Design review of the part shown in the three views and the two pictorial views. Dimensions are in mm from the part's minimum x, y and z. A direction names the side the tool comes from. Give positions to 0.01 mm unless a question says otherwise; leave off trailing zeros. Loops run counter-clockwise (first coordinate to the right, second up) from the corner with the lowest first, then second, coordinate; pieces in that order, holes last. Notation, with made-up numbers: (79.25, 15) - (93.25, 15) arc R36 cw to (93.25, 49) - close; hole circle Ø11 at (-10, -25.5). An arc over 180 degrees is marked (long way). Return JSON: item names as keys, results as strings. Group by question number.
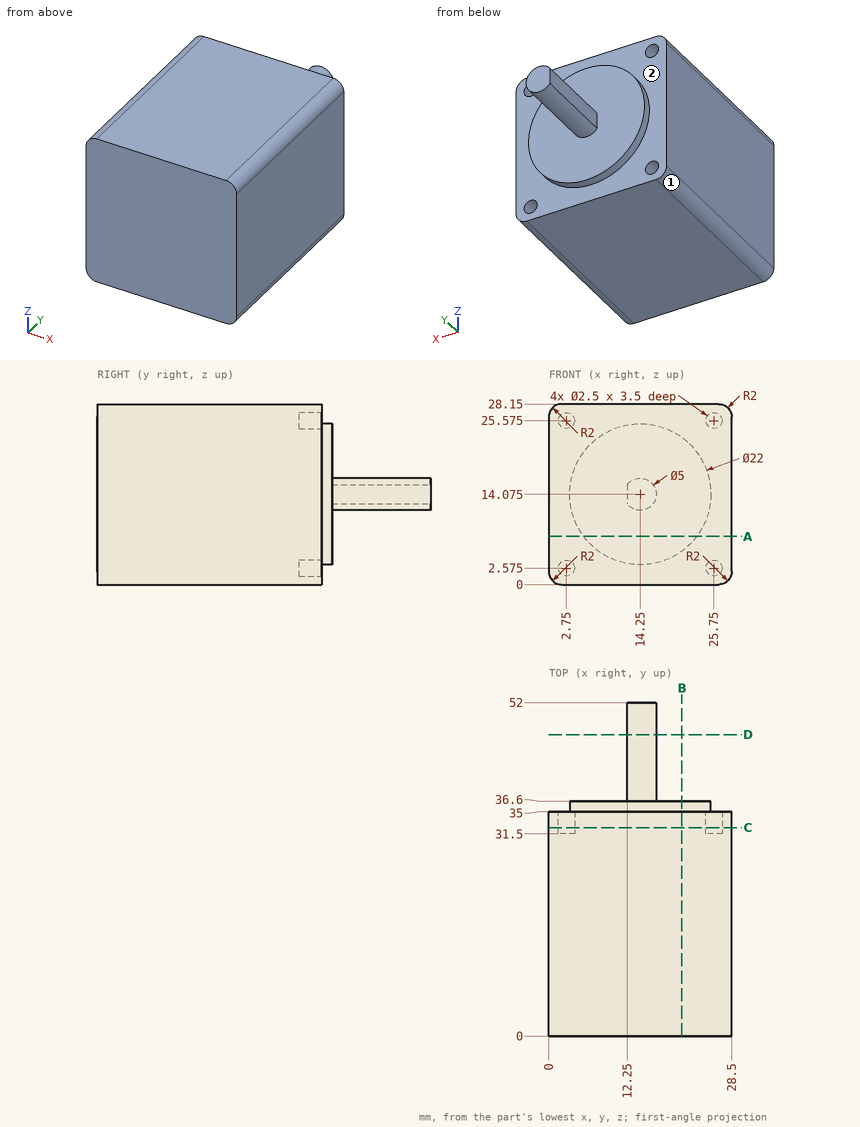
Item 1: For P1, Ø2, axis at x = 25, z = 26, coming from the +Y side; P2, Ø1.5, axis at y = 47, z = 14.5, coming from the -X side, all flat-tipped, find the tip position at first contact; note any pin that passes through.
Item 2: Take a section at A-A (z = 7.5). State the section outline as (x, y) points.
Item 3: For L1, parallel to Z at x = 2.75, y = 34.1 (3 decimals); L2, parallel to Z at x = 16.25, y = 47.5 (3 decimals); L3, parallel to Y at x = 19, z = 13.5, list the stretches that pass through material, from the lowest coordinate up. Write a range as from..to.
Item 4: Take a section at D-D (y = 47). State the section outline as (x, z) points (3 decimals).
Item 5: Take a section at C-C (y = 32.5). State the section outline as (x, z) points (3 decimals), then the cut area to 3 significant figures.
Item 6: Tool access review of the marked faces 1 and 2: name each direction out of +Z, -Z, +X, -X, +Y, -Y from which nothing blocks a thin tool from reaching the whole face with its end or side.
Item 7: Take a section at B-B (x = 20.75). State the section outline as (y, z) points, then the cut area to 3 significant figures.
Check sheet entries:
{
 "1": {"P1": "stops at y = 35", "P2": "stops at x = 12.25"},
 "2": {"outline": "(0, 0) - (28.5, 0) - (28.5, 35) - (23.07, 35) - (23.07, 36.6) - (5.43, 36.6) - (5.43, 35) - (0, 35) - close"},
 "3": {"L1": "z = 0..1.325, 3.825..24.325, 26.825..28.15", "L2": "z = 12.575..15.575", "L3": "y = 0..36.6"},
 "4": {"outline": "(12.25, 12.575) arc R2.5 ccw (long way) to (12.25, 15.575) - close"},
 "5": {"outline": "(0, 2) arc R2 ccw to (2, 0) - (26.5, 0) arc R2 ccw to (28.5, 2) - (28.5, 26.15) arc R2 ccw to (26.5, 28.15) - (2, 28.15) arc R2 ccw to (0, 26.15) - close; hole circle Ø2.5 at (2.75, 2.575); hole circle Ø2.5 at (2.75, 25.575); hole circle Ø2.5 at (25.75, 2.575); hole circle Ø2.5 at (25.75, 25.575)", "area": "779 mm^2"},
 "6": {"face 1": "-Z, -X, +Y, -Y", "face 2": "+Y"},
 "7": {"outline": "(0, 0) - (35, 0) - (35, 5.2) - (36.6, 5.2) - (36.6, 22.95) - (35, 22.95) - (35, 28.15) - (0, 28.15) - close", "area": "1,010 mm^2"}
}
